Part print with two shaded views. Sizes in mm from the minimum x, y, z corner. A direction names the side the tool comes from. Round coordinates to 2 decimals unless told otherwise and drop trailing zeros. Loops run counter-clockwise (first coordinate to the right, second up) from the corner with the lowest first, then second, coordinate; pieces in that order, holes last. Notation, with made-up numbers: (3.25, 43) -> (48.25, 43) arc R17 cw to (48.25, 62) -> close; hole circle Ø11 at (75, 78). An arc over 180 degrees is marked (long way). Use a Markdown table: item, result. Add a question column.
Item 1: Two-plate mould, pull along Y, no slides. Class the marked faces 4, 5 and 6: pulls with the +Y half, pulls with the -Y half, needs draft (parallel to the pull), parting line crosses it, or undercut.
Item 2: Cut at D-D, the plane y = 12. List the corners of the cut face in (x, z).
Item 3: Cut at B-B, the plane y = 20.5. List the corners of the cut face in (x, z), plus the area to 3 significant figures.
Item 4: Which spindle directions (+Z, -Z, +X, -X, +Y, -Y) get a long thin tool onto all of the face, cutting with end or side? Do the marked faces 1, 2 and 3. Say none if no direction does.
Item 5: Cut at A-A, the plane z = 12. List the corners of the cut face in (x, y).
Item 6: Probe line 1 (Z direction, x = 11.5, y = 4); line 2 (Z direction, x = 15.5, y = 11.25); line 3 (Y direction, x = 3, z = 21.5). List the from-to ranges inside material, lowest first. Write a range as [from, to].
Item 7: Cut at C-C, the plane x = 30. List the corners of the cut face in (y, z).
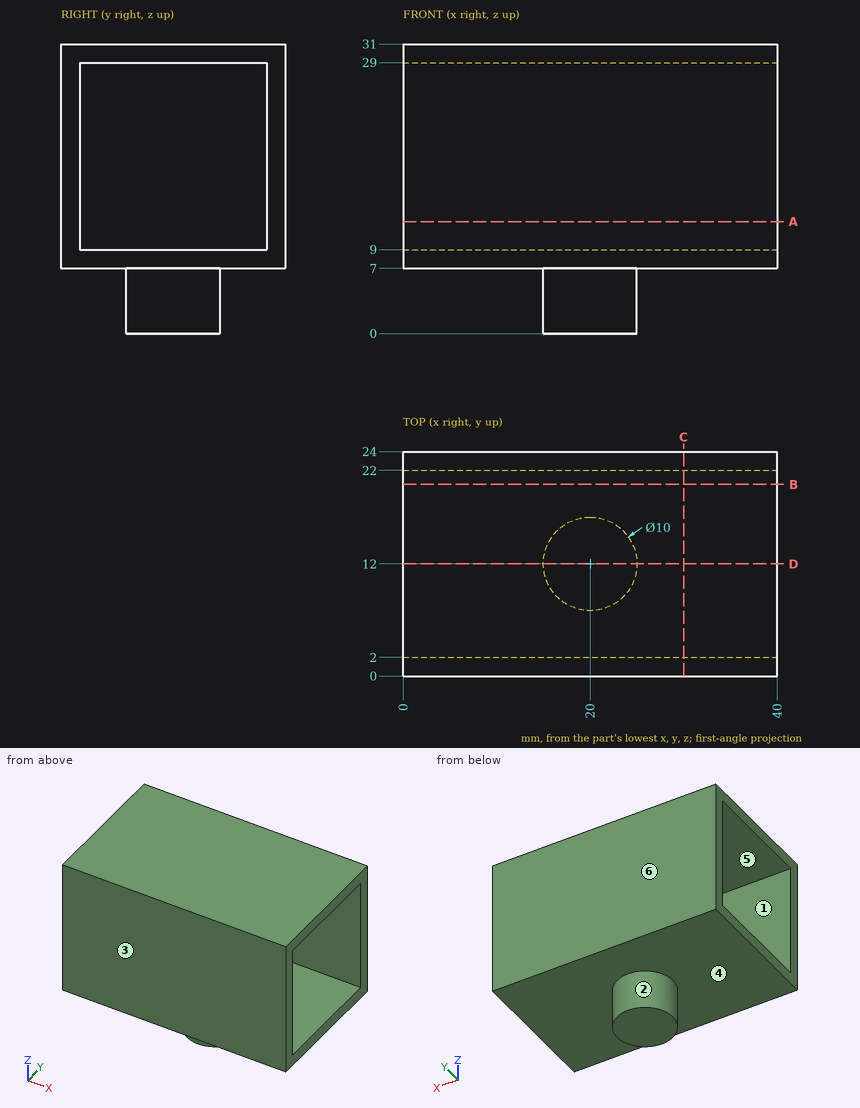
A:
| question | item | result |
|---|---|---|
| 1 | face 4 | needs draft |
| 1 | face 5 | undercut |
| 1 | face 6 | pulls with the +Y half |
| 2 | outline | (0, 7) -> (15, 7) -> (15, 0) -> (25, 0) -> (25, 7) -> (40, 7) -> (40, 9) -> (0, 9) -> close; (0, 29) -> (40, 29) -> (40, 31) -> (0, 31) -> close |
| 3 | outline | (0, 7) -> (40, 7) -> (40, 9) -> (0, 9) -> close; (0, 29) -> (40, 29) -> (40, 31) -> (0, 31) -> close |
| 3 | area | 160 mm^2 |
| 4 | face 1 | +X, -X |
| 4 | face 2 | -Z |
| 4 | face 3 | +Z, -Z, +X, -X, -Y |
| 5 | outline | (0, 0) -> (40, 0) -> (40, 2) -> (0, 2) -> close; (0, 22) -> (40, 22) -> (40, 24) -> (0, 24) -> close |
| 6 | line 1 | z = [7, 9], [29, 31] |
| 6 | line 2 | z = [0, 9], [29, 31] |
| 6 | line 3 | y = [0, 2], [22, 24] |
| 7 | outline | (0, 7) -> (24, 7) -> (24, 31) -> (0, 31) -> close; hole (2, 9) -> (22, 9) -> (22, 29) -> (2, 29) -> close |
